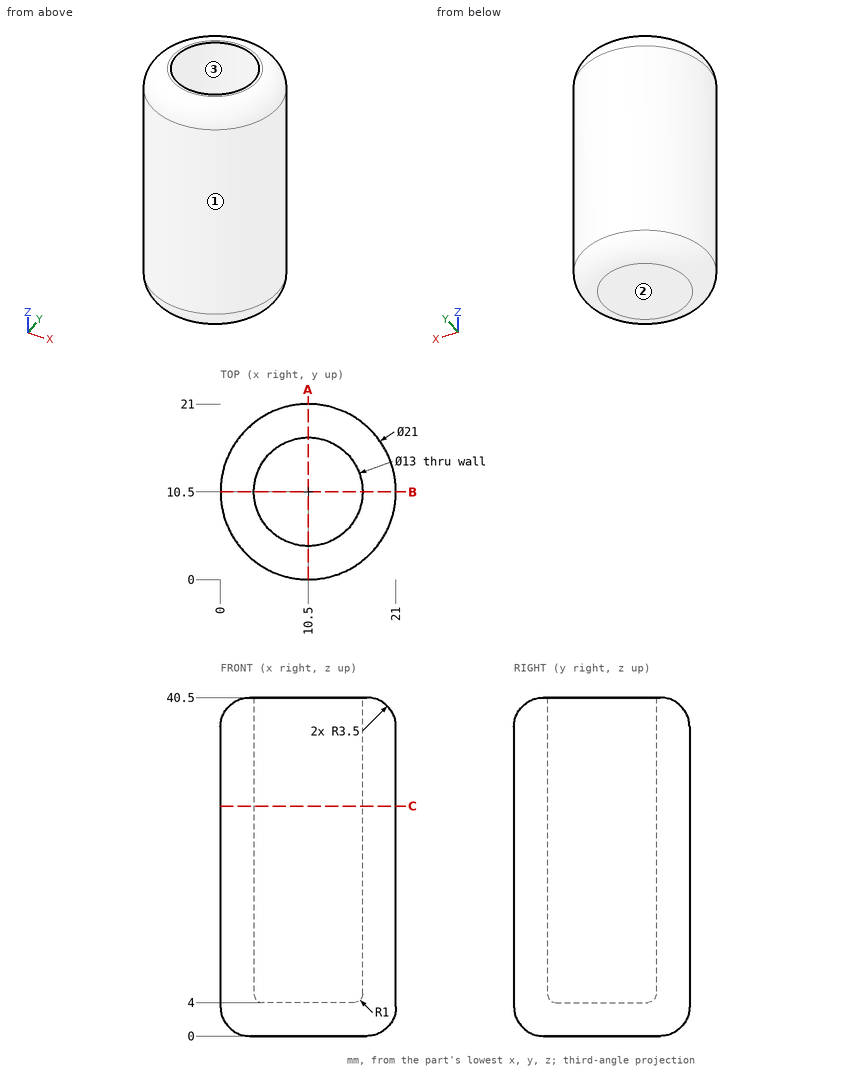
Design review of the part shown in the three views and the two pictorial views. Dimensions are in mm from the part's minimum x, y and z. Coordinates: 2 decimals unless noted, no trailing zeros. Write each loop counter-clockwise with the first axis right and the second up, starting at its lowest first coordinate (ties: lowest second). Pieces come first, ordered by that corner, then holes. Notation, with made-up numbers: (51.5, 21) -> (66.5, 21) arc R20 cw to (66.5, 38) -> close; hole circle Ø10 at (43.25, 33.5). An arc over 180 degrees is marked (long way). Answer in a Markdown table with one row per item.
1. We need section A-A, the plane x = 10.5. State the section outline as (y, z) points, and give its area (3 significant figures).
Answers below:
| item | result |
|---|---|
| outline | (0, 3.5) arc R3.5 ccw to (3.5, 0) -> (17.5, 0) arc R3.5 ccw to (21, 3.5) -> (21, 37) arc R3.5 ccw to (17.5, 40.5) -> (17, 40.5) -> (17, 5) arc R1 cw to (16, 4) -> (5, 4) arc R1 cw to (4, 5) -> (4, 40.5) -> (3.5, 40.5) arc R3.5 ccw to (0, 37) -> close |
| area | 366 mm^2 |
2. Draft analysis for pull direction Y (two halves, no side actions). For the marked faces 1, 2 and 3, state which applies: +Y half, -Y half, draft (parallel to the pull), parting line (faces both ways), or undercut.
Answers below:
| item | result |
|---|---|
| face 1 | parting line |
| face 2 | draft |
| face 3 | undercut |
3. Wall thickness on probe 1 along Y at (x, z) = (10.5, 15); probe 2 along Z at (x, y) = (11.5, 7); probe 3 along Y at (x, z) = (18.75, 14): over which ranges is each line inside the solid? List them lowest first. Write a range as [from, to].
Answers below:
| item | result |
|---|---|
| probe 1 | y = [0, 4], [17, 21] |
| probe 2 | z = [0, 4] |
| probe 3 | y = [4, 17] |
4. We need section C-C, the plane z = 27.5. State the section outline as (x, y) points.
Answers below:
| item | result |
|---|---|
| outline | circle Ø21 at (10.5, 10.5); hole circle Ø13 at (10.5, 10.5) |
5. Clearance check with flat-ended pins moving along their axes: pin 1 Ø1.5 at (x, z) = (15, 19) entering from +Y; pin 2 Ø5 at (x, z) = (10, 5) entering from -Y; pin 3 Ø1 at (y, z) = (4, 18) entering from -X; pin 4 Ø2 at (y, z) = (14.5, 13.5) entering from +X. State where each tip first meets the part, or that it passes through.
Answers below:
| item | result |
|---|---|
| pin 1 | stops at y = 20.31 |
| pin 2 | stops at y = 0 |
| pin 3 | stops at x = 1.88 |
| pin 4 | stops at x = 20.56 |
